Check sheet for the modelled part. Datum: model origin and axes. Units: mm. A direction names the side the tool comes from. Coordinates: 2 decimals unless noted, no trailing zeros. Write each loop counter-clockwise with the first axis right and the second up, starting at its lowest first coordinate (ties: lowest second). Pieces come first, ordered by that corner, then holes. Notation, with made-up numbers: M 6,65.25 L 64,65.25 A18 ccw 64,73.25 Z; hole C 34,62.25 d4. An arc over 180 degrees is marked long. Answer as CSV lines item,"result". Start each with the question number.
Q1. Thickness scan on line 1 along Z through (x, y) = (50.5, 5.5); line 2 along X through (y, z) = (30, 0.5); line 3 along X through (y, z) = (1.5, -2.75). Record the ranges inside material, lowest first. Write a range as from..to.
Q2. Access from +Z, -Z, +X, -X, +Y, -Y to the whole of each face (thin tool, end or side, straight path). Record for faces 1 (the cylindrical face through (-75.95, -2.18, 0.99)), 2 (the cylindrical face through (-35, 0, 4)), 3 (the cylindrical face through (35, 0, -2)).
Q3. Sectioned sample at D-D, the plane x = -1. Record the cut outline in (y, z), then the cut area to 3 significant figures.
Q4. Depth check by flat-ended pin: pin 1 Ø12 at (x, y) = (-8.5, 26) entering from -Z; pin 2 Ø0.6 at (y, z) = (54.5, 1.5) entering from +X; pin 3 Ø4 at (y, z) = (43, -0.5) entering from +X. Enter the tip coordinate at first touch or a pass-through.
Q5. Sectioned sample at B-B, the plane x = 32.5. Record the cut outline in (y, z).
Q6. Sectioned sample at A-A, the plane y = 0. Record the cut outline in (x, z).
Q7. Sectioned sample at C-C, the plane z = -2.5. Record the cut outline in (x, y).
from build123d import *

# Parameters (mm, degrees)
BOSS_EXTRUDE1_DEPTH = 2
SKETCH2_R           = 5
BOSS_EXTRUDE2_DEPTH = 5
SKETCH3_R           = 5
BOSS_EXTRUDE3_DEPTH = 5


with BuildPart() as part:
    # Sketch1 → Boss-Extrude1 (new body)
    with BuildSketch(Plane.XY):
        with BuildLine():
            Line((28.5, 54.486236794), (28.5, 55))
            ThreePointArc((28.5, 55), (26.742640687, 59.242640687), (22.5, 61))
            Line((22.5, 61), (-22.5, 61))
            ThreePointArc((-22.5, 61), (-26.742640687, 59.242640687), (-28.5, 55))
            Line((-28.5, 55), (-28.5, 54.486236794))
            ThreePointArc((-28.5, 54.486236794), (-30.715994747, 48.572078128), (-36.272727273, 45.570307137))
            ThreePointArc((-36.272727273, 45.570307137), (-75.892451058, -3.143713703), (-30, -46))
            Line((-30, -46), (30, -46))
            ThreePointArc((30, -46), (75.892451058, -3.143713703), (36.272727273, 45.570307137))
            ThreePointArc((36.272727273, 45.570307137), (30.715994747, 48.572078128), (28.5, 54.486236794))
        make_face()
    extrude(amount=BOSS_EXTRUDE1_DEPTH)

    # Sketch2 → Boss-Extrude2 (add)
    with BuildSketch(Plane.XY.offset(2)):
        with Locations((-30, 0)):
            Circle(SKETCH2_R)
    extrude(amount=BOSS_EXTRUDE2_DEPTH)

    # Sketch3 → Boss-Extrude3 (add)
    with BuildSketch(Plane(origin=(0, 0, 0), x_dir=(-1, 0, 0), z_dir=(0, 0, -1))):
        with Locations((-30, 0)):
            Circle(SKETCH3_R)
    extrude(amount=BOSS_EXTRUDE3_DEPTH)


solid = part.part
Output:
1,line 1,"z = 0..2"
1,line 2,"x = -64.87..64.87"
1,line 3,"x = 25.23..34.77"
2,face 1,"+Z, -Z, -X"
2,face 2,"+Z"
2,face 3,"-Z"
3,outline,"M -46,0 L 61,0 L 61,2 L -46,2 Z"
3,area,"214 mm^2"
4,pin 1,"stops at z = 0"
4,pin 2,"stops at x = 28.5"
4,pin 3,"stops at x = 50.73"
5,outline,"M -45.93,0 L -4.33,0 L -4.33,-5 L 4.33,-5 L 4.33,0 L 47,0 L 47,2 L -45.93,2 Z"
6,outline,"M -76,0 L 25,0 L 25,-5 L 35,-5 L 35,0 L 76,0 L 76,2 L -25,2 L -25,7 L -35,7 L -35,2 L -76,2 Z"
7,outline,"C 30,0 d10"
